Autodesk Inventor part; units mm, degrees
ref_plane "YZ Plane" through (0, 0, 0) normal (1, 0, 0) x (0, 1, 0)
ref_plane "XZ Plane" through (0, 0, 0) normal (0, 1, 0) x (-1, 0, 0)
ref_plane "XY Plane" through (0, 0, 0) normal (0, 0, 1) x (1, 0, 0)
sketch "Sketch1" plane through (0, 0, 0) normal (0, 1, 0) x (-1, 0, 0)
  line L0 (13.1536, 14.8262) -> (11.1536, 14.8262)
  line L1 (11.1536, 14.8262) -> (11.1536, -15.1738)
  line L2 (11.1536, -15.1738) -> (13.1536, -15.1738)
  line L3 (13.1536, -15.1738) -> (13.1536, 14.8262)
  line L4 (-2.8464, 14.8262) -> (-4.8464, 14.8262)
  line L5 (-4.8464, 14.8262) -> (-4.8464, -15.1738)
  line L6 (-4.8464, -15.1738) -> (-2.8464, -15.1738)
  line L7 (-2.8464, -15.1738) -> (-2.8464, 14.8262)
  line L8 (11.4509, -0.1738) -> (-13.3196, -0.1738)
  line L9 (4.1536, 20.4248) -> (4.1536, -20.4682)
  circle A0 centre (4.1536, -0.1738) radius 5.5
  circle A1 centre (4.1536, -0.1738) radius 7.5
  point P0 (0, 0)
  dimension "d2" = 14
  dimension "d3" = 2
  dimension "d4" = 2
  dimension "d5" = 11
  dimension "d6" = 15
extrude "Extrusion1" add sketch "Sketch1" along normal blind 44 contours L3 L2 L1 A1 L0 | A1 L1 | L1 L8 A0 L9 A1 | L1 A1 L9 A0 L8 | L9 A0 L8 L7 A1 | A1 L8 L5 L4 L7 | L7 L8 A1 | A1 L7 L8 A0 L9 | L7 A1 L8 | A1 L7 L6 L5 L8
sketch "Sketch2" plane through (4.8464, 0, 14.8262) normal (1, 0, 0) x (0, 0, -1)
  line L0 (14.8262, 0) -> (14.8262, 49.2692)
  line L1 (3.5, 48.2793) -> (3.5, -5.9843)
  circle A0 centre (3.5, 40) radius 1.65
  line L2 (0, 0) -> (0, 44)
  line L3 (0, 44) -> (30, 44)
  circle A1 centre (3.5, 35) radius 1.65
  circle A2 centre (3.5, 30) radius 1.65
  circle A3 centre (3.5, 25) radius 1.65
  circle A4 centre (3.5, 20) radius 1.65
  circle A5 centre (3.5, 15) radius 1.65
  circle A6 centre (3.5, 10) radius 1.65
  circle A7 centre (3.5, 5) radius 1.65
  circle A8 centre (26.1523, 40) radius 1.65
  line L4 (29.6523, 0) -> (29.6523, 44)
  circle A9 centre (26.1523, 35) radius 1.65
  circle A10 centre (26.1523, 30) radius 1.65
  circle A11 centre (26.1523, 25) radius 1.65
  circle A12 centre (26.1523, 20) radius 1.65
  circle A13 centre (26.1523, 15) radius 1.65
  circle A14 centre (26.1523, 10) radius 1.65
  circle A15 centre (26.1523, 5) radius 1.65
  circle A16 centre (3.5, 0) radius 1.65
  circle A17 centre (26.1523, 0) radius 1.65
  point P0 (26.1523, 48.2793)
  dimension "d9" = 3.5
  dimension "d10" = 3.3
  dimension "d11" = 4
  dimension "d14" = 5
  dimension "d26" = 5
extrude "Extrusion2" cut sketch "Sketch2" against normal through all contours A0 L1 | A7 L1 | L1 A7 | A6 L1 | L1 A6 | A5 L1 | L1 A5 | A4 L1 | L1 A4 | A3 L1 | L1 A3 | A2 L1 | L1 A2 | A1 L1 | L1 A1 | L1 A0 | A8 | A9 | A10 | A11 | A12 | A13 | A14 | A15
sketch "Sketch3" plane through (0, 0, 0) normal (0, -1, 0) x (1, 0, 0)
  circle A0 centre (-4.1536, -0.1738) radius 5.5
  circle A1 centre (-4.1536, -0.1738) radius 3.5
  point P0 (0, 0)
  dimension "d21" = 2
extrude "Extrusion3" add sketch "Sketch3" against normal blind 1.8
sketch "Sketch4" plane through (4.8464, 0, 14.8262) normal (1, 0, 0) x (0, 0, -1)
  line L0 (14.8262, 0) -> (14.8262, 46.2334)
  line L1 (0, 0) -> (12.3074, 0)
  line L2 (12.8262, 0) -> (16.8262, 0)
  line L3 (16.8262, 0) -> (16.8262, 3)
  line L4 (16.8262, 3) -> (12.8262, 3)
  line L5 (12.8262, 3) -> (12.8262, 0)
  line L6 (12.8262, 41) -> (16.8262, 41)
  line L7 (16.8262, 41) -> (16.8262, 44)
  line L8 (16.8262, 44) -> (12.8262, 44)
  line L9 (12.8262, 44) -> (12.8262, 41)
  dimension "d32" = 4
  dimension "d33" = 3
  dimension "d34" = 4
  dimension "d35" = 3
extrude "Extrusion4" cut sketch "Sketch4" against normal through all
ref_plane "Work Plane1" through (-4.1536, 0, 7.3262) normal (0, 0, 1) x (1, 0, 0)
properties part number "slider-magnet-carrier"
Here's how the part is built. I have some questions about the finished solid (model axes, mm). A direction names the side the tool comes from. Round coordinates to 2 decimals unless told otherwise and drop trailing zeros. Order: outer loops, then holes, each group sorted by start corner. A loop starts at its lowest first (then second) coordinate and runs counter-clockwise, first axis right, second up. Notation, with made-up numbers: (30, 84.5) -> (51, 84.5) arc R17 cw to (51, 88.5) -> close; hole circle Ø5 at (26, -2.5). An arc over 180 degrees is marked (long way). Use CSV: the item, a comma, the result in double quotes.
1. I want a section at C-C on x = -2. List the corners of the cut face in (y, z) for me.
Recorded:
outline,"(0, -7.36) -> (44, -7.36) -> (44, -5.23) -> (1.8, -5.23) -> (1.8, -2.93) -> (0, -2.93) -> close; (0, 2.59) -> (1.8, 2.59) -> (1.8, 4.89) -> (44, 4.89) -> (44, 7.01) -> (0, 7.01) -> close"
2. I'm going to push flat-ended pins straight in: P1, Ø1.2, axis at x = -11, z = -0.5, coming from the -Y side; P2, Ø3, axis at y = 39, z = -12, coming from the +X side; P3, Ø3, axis at x = -5, z = -4, coming from the +Y side. Where does each tip first touch, or does it pass through?
Recorded:
P1,"stops at y = 3"
P2,"stops at x = 4.85"
P3,"stops at y = 1.8"
3. Thinking about a two-plate mould opening in X: for faces 1 (the face through (-4.027, 21.692, 7.325)), 2 (the face through (3.86, 16.39, 10.44)), 3 (the face through (2.846, 22, -9)), 4 (the face through (4.846, 22, 0)), which applies, pulls with the +X half, pulls with the -X half, needs draft (parallel to the pull), parting line crosses it, or undercut?
Recorded:
face 1,"undercut"
face 2,"needs draft"
face 3,"undercut"
face 4,"pulls with the +X half"
4. Which directions (+Z, -Z, +X, -X, +Y, -Y) give clear straight access to the entire face, cutting with the end or side of a thin tool? Please do faces 5 (the face through (-12.14, 36.39, 10.44)), 6 (the face through (3, 1, -2)).
Recorded:
face 5,"+X, -X"
face 6,"+X, -X, -Y"
5. I want a section at A-A on y = 15. Give the number of separate pieces and of enclosed holes in the cut face, and give its area (3 significant figures).
Recorded:
separate pieces,"5"
enclosed holes,"1"
area,"172 mm2"
6. I need wall thicknesses on line 1 along X through (y, z) = (10, 13.75); line 2 along X through (y, z) = (35.5, 5.5); line 3 along X through (y, z) = (35, 3.25). Which ranges of each line are inside material? Lowest first, please.
Recorded:
line 1,"x = -13.15 to -11.15, 2.85 to 4.85"
line 2,"x = -13.15 to -11.15, -9.06 to 0.75, 2.85 to 4.85"
line 3,"x = -13.15 to -11.15, -10.83 to -8.46, 0.15 to 2.52, 2.85 to 4.85"
7. I want a section at B-B on z = 0.5. List the corners of the cut face in (x, y) for me.
Recorded:
outline,"(-13.15, 3) -> (-9.61, 3) -> (-9.61, 41) -> (-13.15, 41) -> close; (1.3, 3) -> (4.85, 3) -> (4.85, 41) -> (1.3, 41) -> close"
